For this review, take the finished solid that the model builds, in its own axes (mm). A direction names the side the tool comes from. Round coordinates to 2 decimals unless told otherwise and drop trailing zeros. Loops run counter-clockwise (first coordinate to the right, second up) from the corner with the lowest first, then second, coordinate; pieces in that order, holes last. Notation, with made-up numbers: (77.5, 35) -> (126.5, 35) arc R20 ccw to (126.5, 42) -> close; hole circle Ø11 at (68.25, 51.5). An arc over 180 degrees is marked (long way). Write each question's results on one line, items separated by ' | '.
```python
from build123d import *

# Parameters (mm, degrees)
ESBO_O1_W                = 250
ESBO_O1_H                = 194
RESSALTO_EXTRUS_O1_DEPTH = 120
ESBO_O2_W                = 215
ESBO_O2_H                = 134
CORTE_EXTRUS_O1_DEPTH    = 5
FILETE1_R                = 15
RESSALTO_EXTRUS_O2_DEPTH = 120
CORTE_EXTRUS_O2_DEPTH    = 0.1
FILETE2_SIZE             = 125
FILETE2_SIZE_2           = 25
ESBO_O7_R                = 4
CORTE_EXTRUS_O3_DEPTH    = 1
ESBO_O8_R                = 2
CORTE_EXTRUS_O4_DEPTH    = 1
ESBO_O9_R                = 0.5
CORTE_EXTRUS_O5_DEPTH    = 1
FILETE4_R                = 12.5
ESBO_O10_R               = 10
CORTE_EXTRUS_O6_DEPTH    = 1
ESBO_O11_R               = 6.5
ESBO_O11_R_2             = 2.5
ESBO_O11_R_3             = 2
ESBO_O11_R_4             = 8
CORTE_EXTRUS_O7_DEPTH    = 1
ESBO_O14_R               = 9
CORTE_EXTRUS_O9_DEPTH    = 2


with BuildPart() as part:
    # Esboço1 → Ressalto-extrusão1 (new body)
    with BuildSketch(Plane.XY):
        Rectangle(ESBO_O1_W, ESBO_O1_H)
    extrude(amount=-RESSALTO_EXTRUS_O1_DEPTH)

    # Esboço2 → Corte-extrusão1 (cut)
    with BuildSketch(Plane.XY):
        with Locations((0, 10)):
            Rectangle(ESBO_O2_W, ESBO_O2_H)
    extrude(amount=-CORTE_EXTRUS_O1_DEPTH, mode=Mode.SUBTRACT)

    # Filete1
    filete1_edges = [part.edges().sort_by_distance(p)[0] for p in [
        (-107.5, 77, -2.5),
        (107.5, 77, -2.5),
        (107.5, -57, -2.5),
        (-107.5, -57, -2.5),
    ]]
    fillet(filete1_edges, radius=FILETE1_R)

    # Esboço3 → Ressalto-extrusão2 (add)
    with BuildSketch(Plane.XY):
        with BuildLine():
            Line((-125, 97), (125, 97))
            ThreePointArc((125, 97), (0, 133), (-125, 97))
        make_face()
    extrude(amount=-RESSALTO_EXTRUS_O2_DEPTH)

    # Esboço4 → Corte-extrusão2 (cut)
    with BuildSketch(Plane.XY):
        with BuildLine():
            Line((117.5, -42), (117.5, 62))
            ThreePointArc((117.5, 62), (110.17766953, 79.67766953), (92.5, 87))
            Line((92.5, 87), (-92.5, 87))
            ThreePointArc((-92.5, 87), (-110.17766953, 79.67766953), (-117.5, 62))
            Line((-117.5, 62), (-117.5, -42))
            ThreePointArc((-117.5, -42), (-110.17766953, -59.67766953), (-92.5, -67))
            Line((-92.5, -67), (92.5, -67))
            ThreePointArc((92.5, -67), (110.17766953, -59.67766953), (117.5, -42))
        make_face()
    extrude(amount=-CORTE_EXTRUS_O2_DEPTH, mode=Mode.SUBTRACT)

    # Filete2
    # a fillet whose section is not a circle: 125, 25 mm, written as the material it takes off along each edge
    with BuildSketch(Plane(origin=(125, -97, 312.5), x_dir=(-1, 0, 0), z_dir=(0, 0, -1))) as filete2_piece_1:
        with BuildLine():
            Bezier((FILETE2_SIZE, 0), (0, 0), (0, FILETE2_SIZE_2), weights=[1, 0.707106781, 1])
            Line((0, FILETE2_SIZE_2), (0, 0))
            Line((0, 0), (FILETE2_SIZE, 0))
        make_face()
    extrude(amount=745, mode=Mode.SUBTRACT)
    with BuildSketch(Plane(origin=(-125, -97, 312.5), x_dir=(1, 0, 0), z_dir=(0, 0, -1))) as filete2_piece_2:
        with BuildLine():
            Bezier((FILETE2_SIZE, 0), (0, 0), (0, -FILETE2_SIZE_2), weights=[1, 0.707106781, 1])
            Line((0, -FILETE2_SIZE_2), (0, 0))
            Line((0, 0), (FILETE2_SIZE, 0))
        make_face()
    extrude(amount=745, mode=Mode.SUBTRACT)

    # Esboço7 → Corte-extrusão3 (cut)
    with BuildSketch(Plane.XY):
        with Locations((0, -82)):
            Circle(ESBO_O7_R)
    extrude(amount=-CORTE_EXTRUS_O3_DEPTH, mode=Mode.SUBTRACT)

    # Esboço8 → Corte-extrusão4 (cut)
    with BuildSketch(Plane.XY.offset(-1)):
        with Locations((0, -82)):
            Circle(ESBO_O8_R)
    extrude(amount=-CORTE_EXTRUS_O4_DEPTH, mode=Mode.SUBTRACT)

    # Esboço9 → Corte-extrusão5 (cut)
    with BuildSketch(Plane.XY):
        with Locations((0, -91.5)):
            Circle(ESBO_O9_R)
        with Locations((0, -93.7)):
            Circle(ESBO_O9_R)
        with Locations((0, -95.9)):
            Circle(ESBO_O9_R)
        with Locations((2.2, -93.7)):
            Circle(ESBO_O9_R)
        with Locations((-2.2, -93.7)):
            Circle(ESBO_O9_R)
        with Locations((40.052268552, -83.754189239)):
            Circle(ESBO_O9_R)
        with Locations((40.052268552, -88.154189239)):
            Circle(ESBO_O9_R)
        with Locations((42.252268552, -85.954189239)):
            Circle(ESBO_O9_R)
        with Locations((37.852268552, -85.954189239)):
            Circle(ESBO_O9_R)
        with Locations((40, -86)):
            Circle(ESBO_O9_R)
        with Locations(Location((-42.252268552, -85.954189239, 0), (0, 0, 180))):
            Circle(ESBO_O9_R)
        with Locations(Location((-40.052268552, -83.754189239, 0), (0, 0, 180))):
            Circle(ESBO_O9_R)
        with Locations(Location((-40, -86, 0), (0, 0, 180))):
            Circle(ESBO_O9_R)
        with Locations(Location((-37.852268552, -85.954189239, 0), (0, 0, 180))):
            Circle(ESBO_O9_R)
        with Locations(Location((-40.052268552, -88.154189239, 0), (0, 0, 180))):
            Circle(ESBO_O9_R)
    extrude(amount=-CORTE_EXTRUS_O5_DEPTH, mode=Mode.SUBTRACT)

    # Filete4
    # the kernel refuses this fillet: 12.5 mm, written as the material it takes off along each edge
    with BuildSketch(Plane(origin=(92.5, 62, -0.1), x_dir=(0, 1, 0), z_dir=(-1, 0, 0))) as filete4_piece_1:
        with BuildLine():
            CenterArc((24.924212815, 12.5), FILETE4_R, 217.445030013, 52.554969987)
            Line((15, 4.9), (15, 0))
            Line((15, 0), (24.924212815, 0))
        make_face()
    revolve(axis=Axis((92.5, 62, -0.1), (0, 0, -1)), revolution_arc=90, mode=Mode.SUBTRACT)
    with BuildSketch(Plane(origin=(-92.5, 77, -0.1), x_dir=(0, 1, 0), z_dir=(1, 0, 0)), Plane(origin=(92.5, -57, -0.1), x_dir=(0, -1, 0), z_dir=(-1, 0, 0))) as filete4_piece_2:
        with BuildLine():
            CenterArc((9.924212815, -12.5), FILETE4_R, 90, 52.554969987)
            Line((0, -4.9), (0, 0))
            Line((0, 0), (9.924212815, 0))
        make_face()
    extrude(amount=185, mode=Mode.SUBTRACT)
    with BuildSketch(Plane(origin=(-92.5, 62, -0.1), x_dir=(-1, 0, 0), z_dir=(0, -1, 0))) as filete4_piece_3:
        with BuildLine():
            CenterArc((24.924212815, 12.5), FILETE4_R, 217.445030013, 52.554969987)
            Line((15, 4.9), (15, 0))
            Line((15, 0), (24.924212815, 0))
        make_face()
    revolve(axis=Axis((-92.5, 62, -0.1), (0, 0, -1)), revolution_arc=90, mode=Mode.SUBTRACT)
    with BuildSketch(Plane(origin=(-107.5, -42, -0.1), x_dir=(-1, 0, 0), z_dir=(0, 1, 0)), Plane(origin=(107.5, 62, -0.1), x_dir=(1, 0, 0), z_dir=(0, -1, 0))) as filete4_piece_4:
        with BuildLine():
            CenterArc((9.924212815, -12.5), FILETE4_R, 90, 52.554969987)
            Line((0, -4.9), (0, 0))
            Line((0, 0), (9.924212815, 0))
        make_face()
    extrude(amount=104, mode=Mode.SUBTRACT)
    with BuildSketch(Plane(origin=(-92.5, -42, -0.1), x_dir=(0, -1, 0), z_dir=(1, 0, 0))) as filete4_piece_5:
        with BuildLine():
            CenterArc((24.924212815, 12.5), FILETE4_R, 217.445030013, 52.554969987)
            Line((15, 4.9), (15, 0))
            Line((15, 0), (24.924212815, 0))
        make_face()
    revolve(axis=Axis((-92.5, -42, -0.1), (0, 0, -1)), revolution_arc=90, mode=Mode.SUBTRACT)
    with BuildSketch(Plane(origin=(92.5, -42, -0.1), x_dir=(1, 0, 0), z_dir=(0, 1, 0))) as filete4_piece_6:
        with BuildLine():
            CenterArc((24.924212815, 12.5), FILETE4_R, 217.445030013, 52.554969987)
            Line((15, 4.9), (15, 0))
            Line((15, 0), (24.924212815, 0))
        make_face()
    revolve(axis=Axis((92.5, -42, -0.1), (0, 0, -1)), revolution_arc=90, mode=Mode.SUBTRACT)

    # Esboço10 → Corte-extrusão6 (cut)
    with BuildSketch(Plane.XY):
        with Locations((-85, 97.924212815)):
            Circle(ESBO_O10_R)
        with BuildLine():
            Line((-40, 113.924212815), (40, 113.924212815))
            ThreePointArc((40, 113.924212815), (49, 104.924212815), (40, 95.924212815))
            Line((40, 95.924212815), (-40, 95.924212815))
            ThreePointArc((-40, 95.924212815), (-49, 104.924212815), (-40, 113.924212815))
        make_face()
    extrude(amount=-CORTE_EXTRUS_O6_DEPTH, mode=Mode.SUBTRACT)

    # Esboço11 → Corte-extrusão7 (cut)
    with BuildSketch(Plane.XY.offset(-1)):
        with Locations((-40, 104.924212815)):
            Circle(ESBO_O11_R)
        with Locations((40, 104.924212815)):
            Circle(ESBO_O11_R)
        with Locations((15, 104.924212815)):
            Circle(ESBO_O11_R)
        with Locations((-25, 110.924212815)):
            Circle(ESBO_O11_R_2)
        with Locations((-25, 98.924212815)):
            Circle(ESBO_O11_R_3)
        with Locations((-85, 97.924212815)):
            Circle(ESBO_O11_R_4)
    extrude(amount=-CORTE_EXTRUS_O7_DEPTH, mode=Mode.SUBTRACT)

    # Esboço14 → Corte-extrusão9 (cut)
    with BuildSketch(Plane.XY):
        with Locations((85, 101)):
            Circle(ESBO_O14_R)
    extrude(amount=-CORTE_EXTRUS_O9_DEPTH, mode=Mode.SUBTRACT)


solid = part.part
```
1. Draft analysis for pull direction X (two halves, no side actions). For faces 1 (the face through (-45.16, 100.97, -1.49)), 2 (the face through (-1, 95, 0)), 3 (the face through (-125, 11, -59)), state which applies: released by +X, released by -X, zero draft, split by the parting line, or undercut.
Values found:
face 1: undercut | face 2: zero draft | face 3: released by -X
2. Consider section A-A (y = 26). State the section outline as (x, z) points.
Values found:
outline: (-125, -120) -> (125, -120) -> (125, 0) -> (117.5, 0) -> (117.5, -0.1) -> (117.42, -0.1) arc R12.5 ccw to (107.5, -5) -> (-107.5, -5) arc R12.5 ccw to (-117.42, -0.1) -> (-117.5, -0.1) -> (-117.5, 0) -> (-125, 0) -> close
3. Tool access review of faces 4 (the face through (-2, 20, -120)), 5 (the face through (-111.962, 9.272, -1.356)): name each direction out of +Z, -Z, +X, -X, +Y, -Y from which nothing blocks a thin tool from reaching the whole face with its end or side.
Values found:
face 4: -Z, +X, -X, +Y, -Y | face 5: +Z
4. To check wall thickness, follow probe 1 along Y at (x, z) = (15, -1.65); probe 2 along Z at (x, y) = (-71.5, -64); probe 3 along Z at (x, y) = (46, -8). State the ranges of each line that lie inside material, in increasing order.
Values found:
probe 1: y = -96.82 to -60.9, 80.9 to 98.42, 111.42 to 132.52 | probe 2: z = -120 to -0.45 | probe 3: z = -120 to -5
5. For pin 1 (10.5 mm diameter, centred on x = 39.5, y = 103.5, fed in from +Z); pin 2 (3 mm diameter, centred on x = 59.5, z = -104.5, fed in from -Y); pin 3 (3 mm diameter, centred on x = -13.5, y = -40, fed in from +Z), all flat-tipped, find the tip position at first contact; note any pin that passes through.
Values found:
pin 1: stops at z = -1 | pin 2: stops at y = -94.15 | pin 3: stops at z = -5
